Geometry check sheet. Reference: the model listing, model coordinates, mm. Coordinates: 2 decimals unless noted, no trailing zeros. Write each loop counter-clockwise with the first axis right and the second up, starting at its lowest first coordinate (ties: lowest second). Pieces come first, ordered by that corner, then holes. Notation, with made-up numbers: (-22, 40.5) - (36, 40.5) arc R34 ccw to (36, 73.5) - close; hole circle Ø8 at (65.25, -6.75). An arc over 180 degrees is marked (long way). Answer as a JSON object with one key per item and string values. Group by question number.
from build123d import *

# Parameters (mm, degrees)
SKETCH2_R           = 57.15
BOSS_EXTRUDE1_DEPTH = 6.35
SKETCH6_R           = 1.7
CUT_EXTRUDE4_DEPTH  = 7.35
CIRPATTERN3_COUNT   = 6


with BuildPart() as part:
    # Sketch2 → Boss-Extrude1 (new body)
    with BuildSketch(Plane.XY):
        Circle(SKETCH2_R)
    extrude(amount=BOSS_EXTRUDE1_DEPTH)

    # Sketch6 → Cut-Extrude4 (cut, through all)
    with BuildSketch(Plane.XY.offset(6.35)):
        with Locations((0, 53.975)):
            Circle(SKETCH6_R)
    cut_extrude4 = extrude(amount=-CUT_EXTRUDE4_DEPTH, mode=Mode.SUBTRACT)

    # CirPattern3: Cut-Extrude4 ×6 about axis
    cirpattern3_axis = Axis((0, 0, 0), (0, 0, 1))
    for i in range(1, CIRPATTERN3_COUNT):
        add(cut_extrude4.rotate(cirpattern3_axis, i * 360 / CIRPATTERN3_COUNT), mode=Mode.SUBTRACT)


solid = part.part
(1) Material ranges on L1, parallel to Y at x = 0, z = 3.75 (3 decimals); L2, parallel to Y at x = -46.5, z = 6; L3, parallel to X at y = 28, z = 4.75, recorded low to high. Write a range as [from, to].
(2) Section check B-B (z = 3). Count the separate pieces of the cut face and the enclosed holes in it, and give its area (3 significant figures).
(3) Section check C-C (y = -15.5). Record the cut outline in (x, z), and give its area (3 significant figures).
(4) Draft check along Y on faces 1 (the face through (-57.095, 2.513, 3.131)), 2 (the face through (-45.173, -27.639, 3.219)), 3 (the face through (-1, 1, 6.35)), 4 (the face through (-46.522, 25.302, 3.219)). Enter one of: +Y half, -Y half, draft (parallel to the pull), parting line (faces both ways), or undercut.
(5) Section check D-D (x = -42.5). Record the cut outline in (y, z), and give its area (3 significant figures).
(6) Section check A-A (x = 0). Record the cut outline in (y, z) (3 decimals), and give its area (3 significant figures).
(7) Gauge pin test, flat ends, axial feed: pin 1 (5.5 mm diameter, centred on x = 46.74, y = 26.99, fed in from -Z); pin 2 (3 mm diameter, centred on y = 45, z = 1, fed in from -X). Record the tip position at first contact, or that the pin passes through.
Conclusion:
{
 "1": {"L1": "y = [-57.15, -55.675], [-52.275, 52.275], [55.675, 57.15]", "L2": "y = [-33.22, -28.67], [-25.31, 25.31], [28.67, 33.22]", "L3": "x = [-49.82, -48.11], [-45.38, 45.38], [48.11, 49.82]"},
 "2": {"separate pieces": "1", "enclosed holes": "6", "area": "10,200 mm^2"},
 "3": {"outline": "(-55.01, 0) - (55.01, 0) - (55.01, 6.35) - (-55.01, 6.35) - close", "area": "699 mm^2"},
 "4": {"face 1": "parting line", "face 2": "undercut", "face 3": "draft", "face 4": "undercut"},
 "5": {"outline": "(-38.21, 0) - (38.21, 0) - (38.21, 6.35) - (-38.21, 6.35) - close", "area": "485 mm^2"},
 "6": {"outline": "(-57.15, 0) - (-55.675, 0) - (-55.675, 6.35) - (-57.15, 6.35) - close; (-52.275, 0) - (52.275, 0) - (52.275, 6.35) - (-52.275, 6.35) - close; (55.675, 0) - (57.15, 0) - (57.15, 6.35) - (55.675, 6.35) - close", "area": "683 mm^2"},
 "7": {"pin 1": "stops at z = 0", "pin 2": "stops at x = -37.07"}
}
